Design review of the part built by this model. Coordinates are the model's own, in mm. A direction names the side the tool comes from. Give positions to 0.01 mm unless a question says otherwise; leave off trailing zeros. Order: outer loops, then holes, each group sorted by start corner. A loop starts at its lowest first (then second) coordinate and runs counter-clockwise, first axis right, second up. Notation, with made-up numbers: M 22,40 L 68,40 A15 cw 68,55 Z; hole C 27.25,19 d10. An arc over 180 degrees is marked long. Put each result on its own line as item: value. Start each with the question number.
from build123d import *

# Parameters (mm, degrees)
SKETCH1_W                       = 120
SKETCH1_H                       = 55
BOSS_EXTRUDE1_DEPTH             = 5
BOSS_EXTRUDE2_DEPTH             = 5
BOSS_EXTRUDE2_DEPTH_BACK        = 2
SKETCH2_W                       = 50
SKETCH2_H                       = 120
SKETCH8_R                       = 1.7
CUT_EXTRUDE4_DEPTH              = 5
CBORE_FOR_M3_SBHCS1_D           = 3.4
CBORE_FOR_M3_SBHCS1_DEPTH       = 3.15
CBORE_FOR_M3_SBHCS1_CBORE_D     = 6.7
CBORE_FOR_M3_SBHCS1_CBORE_DEPTH = 1.65
CBORE_FOR_M3_SBHCS1_TIP         = 1.021463052
CBORE_FOR_M3_SBHCS2_D           = 3.4
CBORE_FOR_M3_SBHCS2_DEPTH       = 3.15
CBORE_FOR_M3_SBHCS2_CBORE_D     = 6.7
CBORE_FOR_M3_SBHCS2_CBORE_DEPTH = 1.65
CBORE_FOR_M3_SBHCS2_TIP         = 1.021463052
CBORE_FOR_M3_SBHCS3_D           = 3.4
CBORE_FOR_M3_SBHCS3_DEPTH       = 3.15
CBORE_FOR_M3_SBHCS3_CBORE_D     = 6.7
CBORE_FOR_M3_SBHCS3_CBORE_DEPTH = 1.65
CBORE_FOR_M3_SBHCS3_TIP         = 1.021463052
CBORE_FOR_M3_SBHCS4_D           = 3.4
CBORE_FOR_M3_SBHCS4_DEPTH       = 3.15
CBORE_FOR_M3_SBHCS4_CBORE_D     = 6.7
CBORE_FOR_M3_SBHCS4_CBORE_DEPTH = 1.65
CBORE_FOR_M3_SBHCS4_TIP         = 1.021463052
SKETCH13_R                      = 3.25
CUT_EXTRUDE5_DEPTH              = 7
SKETCH14_R                      = 1.7
CUT_EXTRUDE6_DEPTH              = 7
SKETCH16_R                      = 1.7
CUT_EXTRUDE8_DEPTH              = 7
CUT_EXTRUDE9_DEPTH              = 2.6


with BuildPart() as part:
    # Sketch1 → Boss-Extrude1 (new body)
    with BuildSketch(Plane.YZ):
        Rectangle(SKETCH1_W, SKETCH1_H)
    extrude(amount=BOSS_EXTRUDE1_DEPTH)

    # Sketch2 → Boss-Extrude2 (add, two sides: drawn at the far end of the back side and taken through both)
    with BuildSketch(Plane(origin=(0, 0, 12.5), x_dir=(-1, 0, 0), z_dir=(0, 0, -1)).offset(-BOSS_EXTRUDE2_DEPTH_BACK)):
        with Locations((-30, 0)):
            Rectangle(SKETCH2_W, SKETCH2_H)
    extrude(amount=BOSS_EXTRUDE2_DEPTH + BOSS_EXTRUDE2_DEPTH_BACK)

    # Sketch8 → Cut-Extrude4 (cut)
    with BuildSketch(Plane.YZ.offset(5)):
        with Locations(Location((-55, 22.5, 0), (0, 0, 270))):
            Circle(SKETCH8_R)
        with Locations(Location((-55, -22.5, 0), (0, 0, 270))):
            Circle(SKETCH8_R)
        with Locations(Location((55, 22.5, 0), (0, 0, 270))):
            Circle(SKETCH8_R)
        with Locations(Location((55, -22.5, 0), (0, 0, 270))):
            Circle(SKETCH8_R)
    extrude(amount=-CUT_EXTRUDE4_DEPTH, mode=Mode.SUBTRACT)

    # CBORE for M3 SBHCS1
    with Locations(Plane(origin=(5, 55, -22.5), x_dir=(0, 0, 1), z_dir=(1, 0, 0))):
        with Locations((0, 0)):
            CounterBoreHole(CBORE_FOR_M3_SBHCS1_D / 2, CBORE_FOR_M3_SBHCS1_CBORE_D / 2, CBORE_FOR_M3_SBHCS1_CBORE_DEPTH, depth=CBORE_FOR_M3_SBHCS1_DEPTH)
            with Locations((0, 0, -(CBORE_FOR_M3_SBHCS1_DEPTH + CBORE_FOR_M3_SBHCS1_TIP / 2))):  # 118° drill point
                Cone(0, CBORE_FOR_M3_SBHCS1_D / 2, CBORE_FOR_M3_SBHCS1_TIP, mode=Mode.SUBTRACT)

    # CBORE for M3 SBHCS2
    with Locations(Plane(origin=(5, 55, 22.5), x_dir=(0, 0, 1), z_dir=(1, 0, 0))):
        with Locations((0, 0)):
            CounterBoreHole(CBORE_FOR_M3_SBHCS2_D / 2, CBORE_FOR_M3_SBHCS2_CBORE_D / 2, CBORE_FOR_M3_SBHCS2_CBORE_DEPTH, depth=CBORE_FOR_M3_SBHCS2_DEPTH)
            with Locations((0, 0, -(CBORE_FOR_M3_SBHCS2_DEPTH + CBORE_FOR_M3_SBHCS2_TIP / 2))):  # 118° drill point
                Cone(0, CBORE_FOR_M3_SBHCS2_D / 2, CBORE_FOR_M3_SBHCS2_TIP, mode=Mode.SUBTRACT)

    # CBORE for M3 SBHCS3
    with Locations(Plane(origin=(5, -55, -22.5), x_dir=(0, 0, 1), z_dir=(1, 0, 0))):
        with Locations((0, 0)):
            CounterBoreHole(CBORE_FOR_M3_SBHCS3_D / 2, CBORE_FOR_M3_SBHCS3_CBORE_D / 2, CBORE_FOR_M3_SBHCS3_CBORE_DEPTH, depth=CBORE_FOR_M3_SBHCS3_DEPTH)
            with Locations((0, 0, -(CBORE_FOR_M3_SBHCS3_DEPTH + CBORE_FOR_M3_SBHCS3_TIP / 2))):  # 118° drill point
                Cone(0, CBORE_FOR_M3_SBHCS3_D / 2, CBORE_FOR_M3_SBHCS3_TIP, mode=Mode.SUBTRACT)

    # CBORE for M3 SBHCS4
    with Locations(Plane(origin=(5, -55, 22.5), x_dir=(0, 0, 1), z_dir=(1, 0, 0))):
        with Locations((0, 0)):
            CounterBoreHole(CBORE_FOR_M3_SBHCS4_D / 2, CBORE_FOR_M3_SBHCS4_CBORE_D / 2, CBORE_FOR_M3_SBHCS4_CBORE_DEPTH, depth=CBORE_FOR_M3_SBHCS4_DEPTH)
            with Locations((0, 0, -(CBORE_FOR_M3_SBHCS4_DEPTH + CBORE_FOR_M3_SBHCS4_TIP / 2))):  # 118° drill point
                Cone(0, CBORE_FOR_M3_SBHCS4_D / 2, CBORE_FOR_M3_SBHCS4_TIP, mode=Mode.SUBTRACT)

    # Sketch13 → Cut-Extrude5 (cut)
    with BuildSketch(Plane(origin=(0, 0, 7.5), x_dir=(1, 0, 0), z_dir=(0, 0, -1))):
        with Locations(Location((34.29, 19.4, 0), (0, 0, 270))):
            Circle(SKETCH13_R)
    extrude(amount=-CUT_EXTRUDE5_DEPTH, mode=Mode.SUBTRACT)

    # Sketch14 → Cut-Extrude6 (cut)
    with BuildSketch(Plane(origin=(0, 0, 7.5), x_dir=(1, 0, 0), z_dir=(0, 0, -1))):
        with Locations(Location((11, -55, 0), (0, 0, 270))):
            Circle(SKETCH14_R)
        with Locations(Location((11, 55, 0), (0, 0, 90))):
            Circle(SKETCH14_R)
    extrude(amount=-CUT_EXTRUDE6_DEPTH, mode=Mode.SUBTRACT)

    # Sketch16 → Cut-Extrude8 (cut)
    with BuildSketch(Plane(origin=(0, 0, 7.5), x_dir=(1, 0, 0), z_dir=(0, 0, -1))):
        with Locations(Location((49, -4, 0), (0, 0, 270))):
            Circle(SKETCH16_R)
    extrude(amount=-CUT_EXTRUDE8_DEPTH, mode=Mode.SUBTRACT)

    # Sketch17 → Cut-Extrude9 (cut)
    with BuildSketch(Plane.XY.offset(14.5)):
        Polygon((7.709103466, 55), (9.354551733, 52.15), (12.645448267, 52.15), (14.290896534, 55), (12.645448267, 57.85), (9.354551733, 57.85), align=None)
        Polygon((46.15, 2.354551733), (49, 0.709103466), (51.85, 2.354551733), (51.85, 5.645448267), (49, 7.290896534), (46.15, 5.645448267), align=None)
        Polygon((7.709108837, -54.9940543), (9.349405291, -57.847022499), (12.640296454, -57.852968198), (14.290891163, -55.0059457), (12.650594709, -52.152977501), (9.359703546, -52.147031802), align=None)
    extrude(amount=-CUT_EXTRUDE9_DEPTH, mode=Mode.SUBTRACT)


solid = part.part
1. Machinability: for faces 1 (the cylindrical face through (31.407, -17.9, 10.951)), 2 (the flat face through (8.54, 56.44, 13.22)), 3 (the cylindrical face through (4.19, -51.73, 21.77)), which of the approach directions +Z, -Z, +X, -X, +Y, -Y give a long, thin tool a straight path to every point of the face, cutting with its end or side? Answer none if there is none.
2. Consider section D-D on y = 50.5. Give the boundary of the cut face in (x, z), then the cut area to 3 significant figures.
3. To check wall thickness, follow probe 1 along Z at (x, y) = (4.4, -55); probe 2 along X at (y, z) = (-19, 12); probe 3 along X at (y, z) = (4, 10). State the ranges of each line that lie inside material, in increasing order.
4. Consider section C-C on z = -22.5. Give the boundary of the cut face in (x, y), then the cut area to 3 significant figures.
5. The part is to be moulded in two halves that separate along Y. For faces 4 (the flat face through (17, 60, 8)), 5 (the flat face through (30, 1, 7.5)), 6 (the flat face through (47.595, 6.48, 13.218)), say which applies: +Y half, -Y half, draft (parallel to the pull), parting line (faces both ways), or undercut.
6. Insertion check: pin 1 (2 mm diameter, centred on x = 11, y = -42, fed in from +Z); pin 2 (4 mm diameter, centred on y = 55, z = 22.5, fed in from +X); pin 3 (4.5 mm diameter, centred on x = 11, y = -55, fed in from +Z). Each pin has a flat end and moves straight along its axis. Give the tip position at first contact, or say it passes through.
7. Consider section B-B on x = 11. Give the boundary of the cut face in (y, z), then the cut area to 3 significant figures.
8. Consider section A-A on y = -19.4. Give the boundary of the cut face in (x, z), then the cut area to 4 significant figures.
Returned:
1. face 1: +Z, -Z
1. face 2: +Z
1. face 3: +X
2. outline: M 0,-27.5 L 5,-27.5 L 5,7.5 L 55,7.5 L 55,14.5 L 5,14.5 L 5,27.5 L 0,27.5 Z
2. area: 625 mm2
3. probe 1: z = -27.5 to -25.85, -19.15 to 19.15, 25.85 to 27.5
3. probe 2: x = 0 to 31.06, 37.52 to 55
3. probe 3: x = 0 to 47.3, 50.7 to 55
4. outline: M 0,-60 L 5,-60 L 5,-58.35 L 3.35,-58.35 L 3.35,-56.7 L 0,-56.7 Z; M 0,-53.3 L 3.35,-53.3 L 3.35,-51.65 L 5,-51.65 L 5,51.65 L 3.35,51.65 L 3.35,53.3 L 0,53.3 Z; M 0,56.7 L 3.35,56.7 L 3.35,58.35 L 5,58.35 L 5,60 L 0,60 Z
4. area: 555 mm2
5. face 4: +Y half
5. face 5: draft
5. face 6: undercut
6. pin 1: stops at z = 14.5
6. pin 2: stops at x = 3.35
6. pin 3: stops at z = 11.9
7. outline: M -60,7.5 L -56.7,7.5 L -56.7,11.9 L -57.85,11.9 L -57.85,14.5 L -60,14.5 Z; M -53.3,7.5 L 53.3,7.5 L 53.3,11.9 L 52.15,11.9 L 52.15,14.5 L -52.15,14.5 L -52.15,11.9 L -53.3,11.9 Z; M 56.7,7.5 L 60,7.5 L 60,14.5 L 57.85,14.5 L 57.85,11.9 L 56.7,11.9 Z
7. area: 780 mm2
8. outline: M 0,-27.5 L 5,-27.5 L 5,7.5 L 31.04,7.5 L 31.04,14.5 L 5,14.5 L 5,27.5 L 0,27.5 Z; M 37.54,7.5 L 55,7.5 L 55,14.5 L 37.54,14.5 Z
8. area: 579.5 mm2
